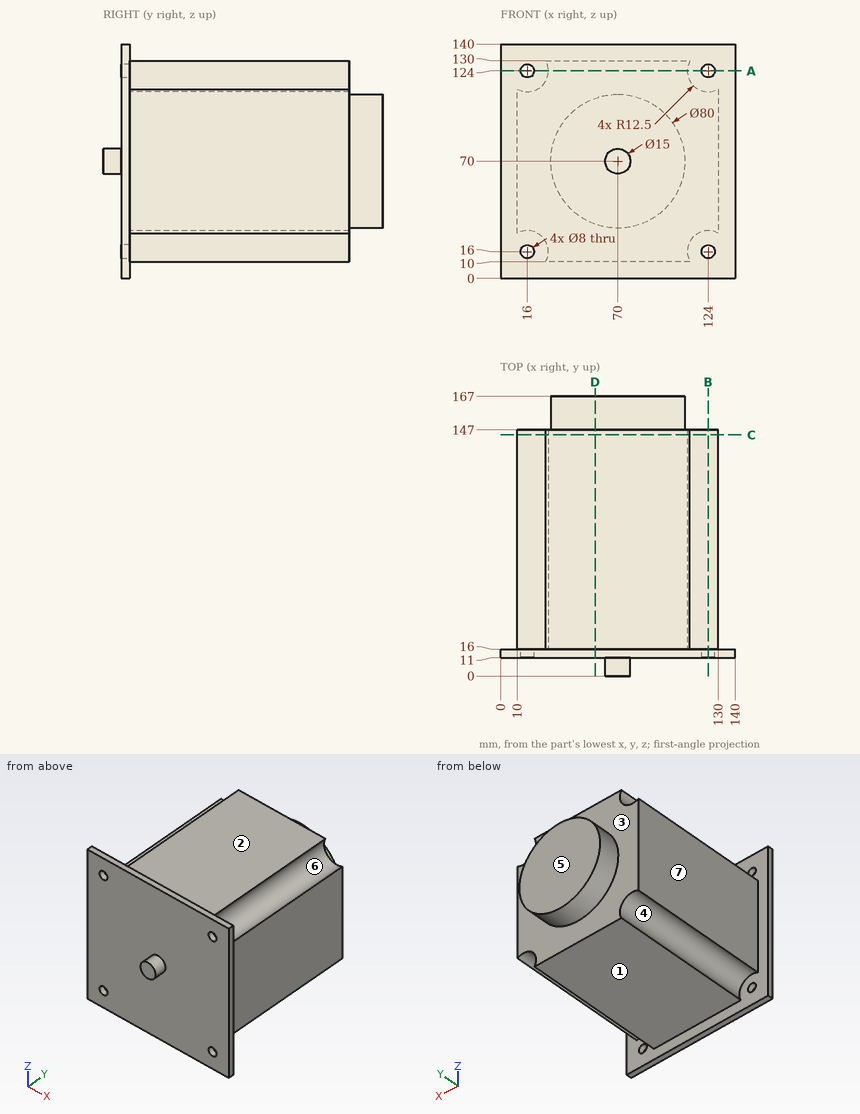
Design review of the part shown in the three views and the two pictorial views. Dimensions are in mm from the part's minimum x, y and z. A direction names the side the tool comes from. Give positions to 0.01 mm unless a question says otherwise; leave off trailing zeros. Order: outer loops, then holes, each group sorted by start corner. A loop starts at its lowest first (then second) coordinate and runs counter-clockwise, first axis right, second up. Notation, with made-up numbers: M 39,-4 L 91,-4 A25 ccw 91,19 Z; hole C 72.5,58 d2. An arc over 180 degrees is marked long. Answer in a Markdown table with one row per item. Add a question column.
(1) Mouldability with a two-part tool opening along X and no side actions: class the marked faces 4, 5, 6 and 7 as +X half, -X half, draft (parallel to the pull), parting line (faces both ways), or undercut.
(2) Consider section A-A on z = 124. State the section outline as (x, y) points.
(3) Consider section B-B on x = 124. State the section outline as (y, z) points, and give its area (3 significant figures).
(4) Wall thickness on probe 1 along X at (y, z) = (12, 16); probe 2 along X at (y, z) = (106, 103.5); probe 3 along Y at (x, z) = (19, 129): over which ranges is each line inside the solid? List them lowest first. Write a range as [from, to].
(5) Consider section D-D on x = 56.5. State the section outline as (y, z) points.
(6) For pin 1 (3 mm diameter, centred on x = 100.5, y = 31, fed in from -Z); pin 2 (5 mm diameter, centred on y = 58, z = 103.5, fed in from +X); pin 3 (5 mm diameter, centred on x = 71, y = 139, fed in from +Z); pin 4 (8 mm diameter, centred on x = 59, y = 18, fed in from -Z), all flat-tipped, find the tip position at first contact; note any pin that passes through.
(7) For the marked faces 1, 2 and 3, list the 3-axis set-ups (+Z, -Z, +X, -X, +Y, -Y) from which the entire face can be reached by the end or side of a thin tool; tool diameter is ignored.
(8) Consider section C-C on y = 144. State the section outline as (x, z) points, and give its area (3 significant figures).
Evaluation:
| question | item | result |
|---|---|---|
| 1 | face 4 | undercut |
| 1 | face 5 | draft |
| 1 | face 6 | undercut |
| 1 | face 7 | -X half |
| 2 | outline | M 0,11 L 12,11 L 12,16 L 0,16 Z; M 20,11 L 120,11 L 120,16 L 111.5,16 L 111.5,147 L 28.5,147 L 28.5,16 L 20,16 Z; M 128,11 L 140,11 L 140,16 L 128,16 Z |
| 3 | outline | M 11,0 L 16,0 L 16,12 L 11,12 Z; M 11,20 L 16,20 L 16,28.5 L 147,28.5 L 147,111.5 L 16,111.5 L 16,120 L 11,120 Z; M 11,128 L 16,128 L 16,140 L 11,140 Z |
| 3 | area | 11,500 mm^2 |
| 4 | probe 1 | x = [0, 12], [20, 120], [128, 140] |
| 4 | probe 2 | x = [10, 130] |
| 4 | probe 3 | y = [11, 16] |
| 5 | outline | M 11,0 L 16,0 L 16,10 L 147,10 L 147,32.35 L 167,32.35 L 167,107.65 L 147,107.65 L 147,130 L 16,130 L 16,140 L 11,140 Z |
| 6 | pin 1 | stops at z = 10 |
| 6 | pin 2 | stops at x = 130 |
| 6 | pin 3 | stops at z = 130 |
| 6 | pin 4 | stops at z = 0 |
| 7 | face 1 | -Z, +X, -X, +Y |
| 7 | face 2 | +Z, +X, -X, +Y |
| 7 | face 3 | +Y |
| 8 | outline | M 10,26.97 A12.5 cw 26.97,10 L 113.03,10 A12.5 cw 130,26.97 L 130,113.03 A12.5 cw 113.03,130 L 26.97,130 A12.5 cw 10,113.03 Z |
| 8 | area | 13,200 mm^2 |
